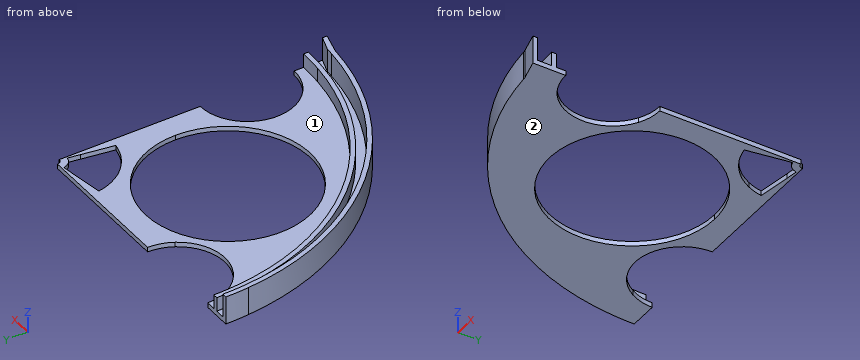
```python
from build123d import *

# Parameters (mm, degrees)
F1_DEPTH = 2.54
F2_DEPTH = 10.16
F3_DEPTH = 2.54
F4_DEPTH = 15.24


with BuildPart() as f1:
    # F0 (on Top) → F1 (new body)
    with BuildSketch(Plane.XY):
        with BuildLine():
            ThreePointArc((-12.7, -134.0196045361), (-6.3570919986, -134.4698173618), (0, -134.62))
            Line((0, -134.62), (0, -129.54))
            ThreePointArc((0, -129.54), (-6.5740037456, -128.6745159877), (-12.7, -126.1370452561))
            Line((-12.7, -126.1370452561), (-12.7, -134.0196045361))
        make_face()
        with BuildLine():
            ThreePointArc((-134.0196045361, -12.7), (-95.1907148833, -95.1907148833), (-12.7, -134.0196045361))
            Line((-12.7, -134.0196045361), (-12.7, -126.1370452561))
            ThreePointArc((-12.7, -126.1370452561), (-25.4, -104.14), (-12.7, -82.1429547439))
            Line((-12.7, -82.1429547439), (-12.7, -57.15))
            ThreePointArc((-12.7, -57.15), (-88.5808964237, -88.5808964237), (-57.15, -12.7))
            Line((-57.15, -12.7), (-82.1429547439, -12.7))
            ThreePointArc((-82.1429547439, -12.7), (-104.14, -25.4), (-126.1370452561, -12.7))
            Line((-126.1370452561, -12.7), (-134.0196045361, -12.7))
        make_face()
        with BuildLine():
            ThreePointArc((-2.510175815, -0.3880945475), (-2.5325329781, -0.1946194105), (-2.54, 0))
            Line((-2.54, 0), (-6.35, 0))
            ThreePointArc((-6.35, 0), (-6.3313324452, -0.4865485263), (-6.2754395375, -0.9702363687))
            Line((-6.2754395375, -0.9702363687), (-2.510175815, -0.3880945475))
        make_face()
        with BuildLine():
            ThreePointArc((-134.62, 0), (-134.4698173618, -6.3570919986), (-134.0196045361, -12.7))
            Line((-134.0196045361, -12.7), (-126.1370452561, -12.7))
            ThreePointArc((-126.1370452561, -12.7), (-128.6745159877, -6.5740037456), (-129.54, 0))
            Line((-129.54, 0), (-134.62, 0))
        make_face()
        with BuildLine():
            ThreePointArc((-57.15, -12.7), (-25.7191035763, -25.7191035763), (-12.7, -57.15))
            Line((-12.7, -57.15), (-12.7, -27.7081287712))
            ThreePointArc((-12.7, -27.7081287712), (-21.5526146906, -21.5526146906), (-27.7081287712, -12.7))
            Line((-27.7081287712, -12.7), (-57.15, -12.7))
        make_face()
        with BuildLine():
            Line((-30.12210978, -4.6571345698), (-82.1429547439, -12.7))
            Line((-82.1429547439, -12.7), (-57.15, -12.7))
            Line((-57.15, -12.7), (-27.7081287712, -12.7))
            ThreePointArc((-27.7081287712, -12.7), (-29.1934246673, -8.7620977053), (-30.12210978, -4.6571345698))
        make_face()
        with BuildLine():
            Line((-12.7, -57.15), (-12.7, -82.1429547439))
            Line((-12.7, -82.1429547439), (-4.6571345698, -30.12210978))
            ThreePointArc((-4.6571345698, -30.12210978), (-8.7620977053, -29.1934246673), (-12.7, -27.7081287712))
            Line((-12.7, -27.7081287712), (-12.7, -57.15))
        make_face()
        with BuildLine():
            ThreePointArc((-12.7, -82.1429547439), (-6.5740037456, -79.6054840123), (0, -78.74))
            Line((0, -78.74), (0, -30.48))
            ThreePointArc((0, -30.48), (-2.3354329262, -30.3903957369), (-4.6571345698, -30.12210978))
            Line((-4.6571345698, -30.12210978), (-12.7, -82.1429547439))
        make_face()
        with BuildLine():
            ThreePointArc((-4.6571345698, -30.12210978), (-2.3354329262, -30.3903957369), (0, -30.48))
            Line((0, -30.48), (0, -12.7))
            Line((0, -12.7), (-1.9635281017, -12.7))
            Line((-1.9635281017, -12.7), (-4.6571345698, -30.12210978))
        make_face()
        with BuildLine():
            Line((-1.9635281017, -12.7), (0, -12.7))
            Line((0, -12.7), (0, -6.35))
            ThreePointArc((0, -6.35), (-0.4865485263, -6.3313324452), (-0.9702363687, -6.2754395375))
            Line((-0.9702363687, -6.2754395375), (-1.9635281017, -12.7))
        make_face()
        with BuildLine():
            ThreePointArc((-0.9702363687, -6.2754395375), (-0.4865485263, -6.3313324452), (0, -6.35))
            Line((0, -6.35), (0, -2.54))
            ThreePointArc((0, -2.54), (-0.1946194105, -2.5325329781), (-0.3880945475, -2.510175815))
            Line((-0.3880945475, -2.510175815), (-0.9702363687, -6.2754395375))
        make_face()
        with BuildLine():
            Line((-0.9702363687, -6.2754395375), (-0.3880945475, -2.510175815))
            ThreePointArc((-0.3880945475, -2.510175815), (-1.7960512242, -1.7960512242), (-2.510175815, -0.3880945475))
            Line((-2.510175815, -0.3880945475), (-6.2754395375, -0.9702363687))
            ThreePointArc((-6.2754395375, -0.9702363687), (-4.4901280605, -4.4901280605), (-0.9702363687, -6.2754395375))
        make_face()
        with BuildLine():
            ThreePointArc((-30.48, 0), (-30.3903957369, -2.3354329262), (-30.12210978, -4.6571345698))
            Line((-30.12210978, -4.6571345698), (-12.7, -1.9635281017))
            Line((-12.7, -1.9635281017), (-12.7, 0))
            Line((-12.7, 0), (-30.48, 0))
        make_face()
        with BuildLine():
            Line((-12.7, 0), (-12.7, -1.9635281017))
            Line((-12.7, -1.9635281017), (-6.2754395375, -0.9702363687))
            ThreePointArc((-6.2754395375, -0.9702363687), (-6.3313324452, -0.4865485263), (-6.35, 0))
            Line((-6.35, 0), (-12.7, 0))
        make_face()
        with BuildLine():
            ThreePointArc((-78.74, 0), (-79.6054840123, -6.5740037456), (-82.1429547439, -12.7))
            Line((-82.1429547439, -12.7), (-30.12210978, -4.6571345698))
            ThreePointArc((-30.12210978, -4.6571345698), (-30.3903957369, -2.3354329262), (-30.48, 0))
            Line((-30.48, 0), (-78.74, 0))
        make_face()
    extrude(amount=F1_DEPTH)

    # F0 (on Top) → F2 (join)
    with BuildSketch(Plane.XY):
        with BuildLine():
            Line((0, -137.16), (0, -134.62))
            ThreePointArc((0, -134.62), (-6.3570919986, -134.4698173618), (-12.7, -134.0196045361))
            Line((-12.7, -134.0196045361), (-12.7, -136.5707713971))
            ThreePointArc((-12.7, -136.5707713971), (-6.3568307817, -137.0126136617), (0, -137.16))
        make_face()
        with BuildLine():
            Line((-12.7, -136.5707713971), (-12.7, -134.0196045361))
            ThreePointArc((-12.7, -134.0196045361), (-95.1907148833, -95.1907148833), (-134.0196045361, -12.7))
            Line((-134.0196045361, -12.7), (-136.5707713971, -12.7))
            ThreePointArc((-136.5707713971, -12.7), (-96.9867661075, -96.9867661075), (-12.7, -136.5707713971))
        make_face()
        with BuildLine():
            Line((-136.5707713971, -12.7), (-134.0196045361, -12.7))
            ThreePointArc((-134.0196045361, -12.7), (-134.4698173618, -6.3570919986), (-134.62, 0))
            Line((-134.62, 0), (-137.16, 0))
            ThreePointArc((-137.16, 0), (-137.0126136617, -6.3568307817), (-136.5707713971, -12.7))
        make_face()
    extrude(amount=F2_DEPTH)

    # F0 (on Top) → F3 (join)
    with BuildSketch(Plane.XY):
        with BuildLine():
            Line((0, -142.24), (0, -137.16))
            ThreePointArc((0, -137.16), (-6.3568307817, -137.0126136617), (-12.7, -136.5707713971))
            Line((-12.7, -136.5707713971), (-12.7, -141.6719012366))
            ThreePointArc((-12.7, -141.6719012366), (-10.6556073906, -141.8403173683), (-8.6089986235, -141.979233491))
            ThreePointArc((-8.6089986235, -141.979233491), (-4.306473513, -142.1747934265), (0, -142.24))
        make_face()
        with BuildLine():
            Line((0, -144.78), (0, -142.24))
            ThreePointArc((0, -142.24), (-4.306473513, -142.1747934265), (-8.6089986235, -141.979233491))
            Line((-8.6089986235, -141.979233491), (0, -144.78))
        make_face()
        with BuildLine():
            Line((-12.7, -141.6719012366), (-12.7, -136.5707713971))
            ThreePointArc((-12.7, -136.5707713971), (-96.9867661075, -96.9867661075), (-136.5707713971, -12.7))
            Line((-136.5707713971, -12.7), (-141.6719012366, -12.7))
            ThreePointArc((-141.6719012366, -12.7), (-100.578868556, -100.578868556), (-12.7, -141.6719012366))
        make_face()
        with BuildLine():
            Line((-141.6719012366, -12.7), (-136.5707713971, -12.7))
            ThreePointArc((-136.5707713971, -12.7), (-137.0126136617, -6.3568307817), (-137.16, 0))
            Line((-137.16, 0), (-142.24, 0))
            ThreePointArc((-142.24, 0), (-142.0979043334, -6.3563499), (-141.6719012366, -12.7))
        make_face()
    extrude(amount=F3_DEPTH)

    # F0 (on Top) → F4 (join)
    with BuildSketch(Plane.XY):
        with BuildLine():
            ThreePointArc((-8.6089986235, -141.979233491), (-10.6556073906, -141.8403173683), (-12.7, -141.6719012366))
            Line((-12.7, -141.6719012366), (-12.7, -144.2219067964))
            ThreePointArc((-12.7, -144.2219067964), (-12.1332804652, -144.2706896953), (-11.5663736451, -144.3172456801))
            ThreePointArc((-11.5663736451, -144.3172456801), (-5.787813509, -144.6642651617), (0, -144.78))
            Line((0, -144.78), (-8.6089986235, -141.979233491))
        make_face()
        with BuildLine():
            Line((0, -147.32), (0, -144.78))
            ThreePointArc((0, -144.78), (-5.787813509, -144.6642651617), (-11.5663736451, -144.3172456801))
            Line((-11.5663736451, -144.3172456801), (0, -147.32))
        make_face()
        with BuildLine():
            Line((-12.7, -144.2219067964), (-12.7, -141.6719012366))
            ThreePointArc((-12.7, -141.6719012366), (-100.578868556, -100.578868556), (-141.6719012366, -12.7))
            Line((-141.6719012366, -12.7), (-144.2219067964, -12.7))
            ThreePointArc((-144.2219067964, -12.7), (-102.3749197802, -102.3749197802), (-12.7, -144.2219067964))
        make_face()
        with BuildLine():
            Line((-144.2219067964, -12.7), (-141.6719012366, -12.7))
            ThreePointArc((-141.6719012366, -12.7), (-142.0979043334, -6.3563499), (-142.24, 0))
            Line((-142.24, 0), (-144.78, 0))
            ThreePointArc((-144.78, 0), (-144.6404094055, -6.3561283031), (-144.2219067964, -12.7))
        make_face()
    extrude(amount=F4_DEPTH)


solid = f1.part
```
Geometry check sheet. Reference: the model listing, model coordinates, mm. Face numbers are marked on the shaded views. A direction names the side the tool comes from. Coordinates: 2 decimals unless noted, no trailing zeros. Order: outer loops, then holes, each group sorted by start corner. A loop starts at its lowest first (then second) coordinate and runs counter-clockwise, first axis right, second up. Notation, with made-up numbers: (83, -26.5) - (135, -26.5) arc R14 cw to (135, -6.5) - close; hole circle Ø8 at (-29.75, 6.25). An arc over 180 degrees is marked (long way). Use one line per item in the form item = value.
1. Section check D-D (y = -85.5). Record the boundary of the cut face in (x, z).
Here are the results:
outline = (-116.84, 0) - (-91.39, 0) - (-91.39, 2.54) - (-103.98, 2.54) - (-103.98, 10.16) - (-107.25, 10.16) - (-107.25, 2.54) - (-113.67, 2.54) - (-113.67, 15.24) - (-116.84, 15.24) - close; (-22.91, 0) - (-17.25, 0) - (-17.25, 2.54) - (-22.91, 2.54) - close
2. Access from +Z, -Z, +X, -X, +Y, -Y to the whole of each face (thin tool, end or side, straight path). Record for the marked faces 1 and 2.
Here are the results:
face_1 = +Z, +X, +Y
face_2 = -Z, +X, -X, +Y, -Y
3. Scan lines: line 1 (Z direction, x = -35, y = -122.5); line 2 (Y direction, x = -57.15, z = 1.4). Record each from-to range of solid material in increasing order.
Here are the results:
line_1 = 0 to 2.54
line_2 = -133.02 to -101.6, -12.7 to 0
4. Gauge pin test, flat ends, axial feed: pin 1 (5 mm diameter, centred on y = -56, z = 10, fed in from -X); pin 2 (5 mm diameter, centred on x = -119.5, y = -45.5, fed in from -Z); pin 3 (3 mm diameter, centred on x = -112, z = 7, fed in from -Y); pin 4 (3 mm diameter, centred on x = -22.5, z = 12, fed in from -Y). Record the tip position at first contact, or that the pin passes through.
Here are the results:
pin_1 = -134.53
pin_2 = 0
pin_3 = -93.55
pin_4 = -143.25
5. Section check B-B (x = -89). Record the boundary of the cut face in (y, z).
Here are the results:
outline = (-114.19, 0) - (-88.16, 0) - (-88.16, 2.54) - (-101, 2.54) - (-101, 10.16) - (-104.36, 10.16) - (-104.36, 2.54) - (-110.96, 2.54) - (-110.96, 15.24) - (-114.19, 15.24) - close; (-26.14, 0) - (-20.39, 0) - (-20.39, 2.54) - (-26.14, 2.54) - close
6. Section check C-C (y = -17). Record the boundary of the cut face in (x, z), then the cut area to 3 significant figures.
Here are the results:
outline = (-143.78, 0) - (-123.01, 0) - (-123.01, 2.54) - (-133.54, 2.54) - (-133.54, 10.16) - (-136.1, 10.16) - (-136.1, 2.54) - (-141.22, 2.54) - (-141.22, 15.24) - (-143.78, 15.24) - close; (-85.27, 0) - (-76.22, 0) - (-76.22, 2.54) - (-85.27, 2.54) - close; (-38.08, 0) - (-25.3, 0) - (-25.3, 2.54) - (-38.08, 2.54) - close; (-2.63, 0) - (0, 0) - (0, 2.54) - (-2.63, 2.54) - close
area = 167 mm²
7. Section check A-A (z = 7.5). Record the boundary of the cut face in (x, y), then the cut area to 3 significant figures.
Here are the results:
outline = (-144.78, 0) arc R144.78 ccw to (-12.7, -144.22) arc R144.78 ccw to (-11.57, -144.32) - (0, -147.32) - (0, -144.78) - (-8.61, -141.98) arc R142.24 cw to (-142.24, 0) - close; (-137.16, 0) arc R137.16 ccw to (0, -137.16) - (0, -134.62) arc R134.62 cw to (-134.62, 0) - close
area = 1,120 mm²
